```python
from build123d import *

# Parameters (mm, degrees)
SKETCH_1_R             = 13
EXTRUDE_1_DEPTH        = 14
EXTRUDE_2_DEPTH        = 71
SKETCH_3_R             = 13
CUT_EXTRUDE_1_DEPTH    = 402.319595452
PATTERN_LINEAR_1_COUNT = 4
PATTERN_LINEAR_1_PITCH = 80


with BuildPart() as part:
    # 草图1 → 凸台-拉伸1 (new body)
    with BuildSketch(Plane.XY):
        Polygon((71.4349048, -49.703584356), (71.4349048, -264.703584356), (11.4349048, -324.703584356), (-148.5650952, -234.703584356), (-148.5650952, 85.296415644), align=None)
        with Locations((-43.0650952, -212.828584356)):
            Circle(SKETCH_1_R, mode=Mode.SUBTRACT)
        with Locations((10.084011906, -272.621329851)):
            Circle(SKETCH_1_R, mode=Mode.SUBTRACT)
    extrude(amount=EXTRUDE_1_DEPTH)

    # 草图2 → 凸台-拉伸2 (add)
    with BuildSketch(Plane.XY.offset(14)):
        Polygon((-134.5650952, 76.705506553), (-134.5650952, -242.578584356), (-148.5650952, -234.703584356), (-148.5650952, 85.296415644), align=None)
    extrude(amount=EXTRUDE_2_DEPTH)

    # 草图3 → 切除-拉伸1 (cut, through all)
    with BuildSketch(Plane.ZY.offset(148.5650952)):
        with Locations((47, 45.296415644)):
            Circle(SKETCH_3_R)
    cut_extrude_1 = extrude(amount=-CUT_EXTRUDE_1_DEPTH, mode=Mode.SUBTRACT)

    # 阵列(线性)1: 切除-拉伸1 ×4
    with Locations(*[(0, -i * PATTERN_LINEAR_1_PITCH, 0) for i in range(1, PATTERN_LINEAR_1_COUNT)]):
        add(cut_extrude_1, mode=Mode.SUBTRACT)


solid = part.part
```
Can you work these out from the model? Positions are in its coordinate system, mm. A direction names the side the tool comes from. Coordinates: 2 decimals unless noted, no trailing zeros. Loops run counter-clockwise (first coordinate to the right, second up) from the corner with the lowest first, then second, coordinate; pieces in that order, holes last. Notation, with made-up numbers: (52, 13) -> (81, 13) arc R10 cw to (81, 28) -> close; hole circle Ø11 at (4.5, 49). An arc over 180 degrees is marked (long way). Answer as a JSON object with one key per item and string values.
1) Imagine slicing it at A-A (z = 47). Please give me the cut outline in (x, y), then the cut area to 3 significant figures.
Results:
{"outline": "(-148.57, -234.7) -> (-134.57, -242.58) -> (-134.57, -207.7) -> (-148.57, -207.7) -> close; (-148.57, -181.7) -> (-134.57, -181.7) -> (-134.57, -127.7) -> (-148.57, -127.7) -> close; (-148.57, -101.7) -> (-134.57, -101.7) -> (-134.57, -47.7) -> (-148.57, -47.7) -> close; (-148.57, -21.7) -> (-134.57, -21.7) -> (-134.57, 32.3) -> (-148.57, 32.3) -> close; (-148.57, 58.3) -> (-134.57, 58.3) -> (-134.57, 76.71) -> (-148.57, 85.3) -> close", "area": "3,020 mm^2"}
2) For faces 1 (the face through (-91.895, -266.58, 10.82)), 2 (the face through (-134.565, -81, 49)), which set-ups out of +Z, -Z, +X, -X, +Y, -Y let a thin tool reach every point of the face, with its end or its side?
Results:
{"face 1": "+Z, -Z, -X, -Y", "face 2": "+Z, +X, +Y, -Y"}
3) For P1, Ø2, axis at y = -166, z = 27, coming from the +X side; P2, Ø3, axis at x = -75.5, y = -161.5, coming from the -Z side; P3, Ø15.5, axis at y = 45.3, z = 47, coming from the +X side; P4, Ø5, axis at x = -10, z = 11.5, coming from the -Y side, each with a flat end and sliding along its axis, tell me the tip position at first contact or that it passes through.
Results:
{"P1": "stops at x = -134.57", "P2": "stops at z = 0", "P3": "passes through", "P4": "stops at y = -314.05"}
4) Imagine slicing it at C-C (y = -230). Please give me the cut outline in (x, z).
Results:
{"outline": "(-148.57, 0) -> (71.43, 0) -> (71.43, 14) -> (-134.57, 14) -> (-134.57, 85) -> (-148.57, 85) -> close"}
5) Thinking about a two-plate mould opening in Z: for faces 3 (the face through (-141.663, -34.132, 34.013)), 4 (the face through (-30, -121, 14)), 5 (the face through (-148.565, -77, 42)), which applies, pulls with the +Z half, pulls with the -Z half, needs draft (parallel to the pull), parting line crosses it, or undercut?
Results:
{"face 3": "undercut", "face 4": "pulls with the +Z half", "face 5": "needs draft"}
6) If I drill on line 1 (Y direction, x = -138, z = 47); line 2 (Y direction, x = -144, z = 47); line 3 (Z direction, x = 61.5, y = -265.5), over which ranges is the centre line in solid material (lowest first)?
Results:
{"line 1": "y = -240.65 to -207.7, -181.7 to -127.7, -101.7 to -47.7, -21.7 to 32.3, 58.3 to 78.81", "line 2": "y = -237.27 to -207.7, -181.7 to -127.7, -101.7 to -47.7, -21.7 to 32.3, 58.3 to 82.5", "line 3": "z = 0 to 14"}
7) Imagine slicing it at D-D (z = 80). Please give me the cut outline in (x, y).
Results:
{"outline": "(-148.57, -234.7) -> (-134.57, -242.58) -> (-134.57, 76.71) -> (-148.57, 85.3) -> close"}
8) Imagine slicing it at B-B (x = -40). Please give me the cut outline in (y, z).
Results:
{"outline": "(-295.77, 0) -> (-225.46, 0) -> (-225.46, 14) -> (-295.77, 14) -> close; (-200.2, 0) -> (18.68, 0) -> (18.68, 14) -> (-200.2, 14) -> close"}
